Verification items for this drawing (mm, ordinates from the low corner). A direction names the side the tool comes from. Coordinates: 2 decimals unless noted, no trailing zeros. Order: outer loops, then holes, each group sorted by start corner. A loop starts at its lowest first (then second) coordinate and runs counter-clockwise, first axis right, second up. Notation, with made-up numbers: M -9.75,-27 L 5.25,-27 A18 ccw 5.25,8 Z; hole C 28,52.25 d6. An arc over 180 degrees is marked long. Write item = value, one per line.
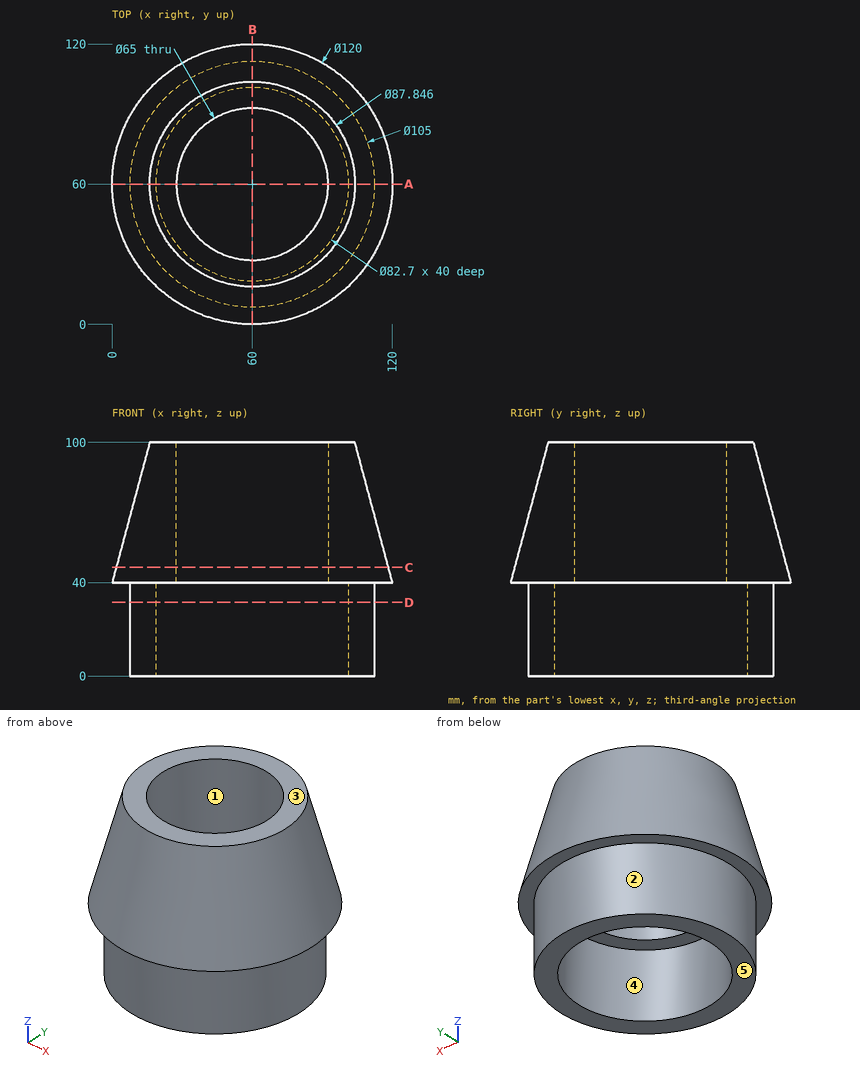
Item 1: Tool access check on the marked faces 4 and 5. Record the directions out of +Z, -Z, +X, -X, +Y, -Y that give a thin tool (end or side, any length) a straight path to the whole face; none if there is none.
Report:
face_4 = -Z
face_5 = -Z, +X, -X, +Y, -Y
Item 2: Scan lines: L1, parallel to Y at x = 60, z = 15; L2, parallel to Y at x = 71, z = 55; L3, parallel to Z at x = 72, y = 97.5. Record each from-to range of solid material in increasing order. Write a range as from..to.
Report:
L1 = 7.5..18.65, 101.35..112.5
L2 = 5.11..29.42, 90.58..114.89
L3 = 40..100
Item 3: Release check for a two-part mould opening along X. For the marked faces 1, 2 and 3 record: pulls with the +X half, pulls with the -X half, needs draft (parallel to the pull), parting line crosses it, or undercut.
Report:
face_1 = undercut
face_2 = parting line crosses it
face_3 = needs draft
Item 4: Sectioned sample at A-A, the plane y = 60. Enter the section's corners in (x, z).
Report:
outline = M 0,40 L 7.5,40 L 7.5,0 L 18.65,0 L 18.65,40 L 27.5,40 L 27.5,100 L 16.08,100 Z; M 92.5,40 L 101.35,40 L 101.35,0 L 112.5,0 L 112.5,40 L 120,40 L 103.92,100 L 92.5,100 Z
Item 5: Sectioned sample at D-D, the plane z = 31.5. Enter the section's corners in (x, y), then the cut area to 3 significant figures.
Report:
outline = C 60,60 d105; hole C 60,60 d82.7
area = 3,290 mm^2
Item 6: Sectioned sample at C-C, the plane z = 46.5. Enter the section's corners in (x, y).
Report:
outline = C 60,60 d116.52; hole C 60,60 d65
Item 7: Gauge pin test, flat ends, axial feed: pin 1 (4 mm diameter, centred on y = 88, z = 15, fed in from +X); pin 2 (3 mm diameter, centred on y = 46, z = 66.5, fed in from -X); pin 3 (8 mm diameter, centred on x = 87.5, z = 85, fed in from -Y). Record the tip position at first contact, or that the pin passes through.
Report:
pin_1 = 105.61
pin_2 = 8.41
pin_3 = 17.9
